```python
from build123d import *

# Parameters (mm, degrees)
SKETCH1_W                       = 9.525
SKETCH1_H                       = 9.525
BOSS_EXTRUDE1_DEPTH             = 9.525
CUT_EXTRUDE2_DEPTH              = 10.525
CUT_EXTRUDE3_DEPTH              = 10.525
F_5_64_0_07813_DIAMETER_HOLE1_D = 1.984502


with BuildPart() as part:
    # Sketch1 → Boss-Extrude1 (new body)
    with BuildSketch(Plane(origin=(0, 0, 0), x_dir=(1, 0, 0), z_dir=(0, 1, 0))):
        with BuildLine():
            Line((-4.138568073, 94.60926025), (4.138568073, 94.60926025))
            ThreePointArc((4.138568073, 94.60926025), (8.245532024, 93.102332324), (10.40323655, 89.29677115))
            Line((10.40323655, 89.29677115), (10.40323655, -5.448440201))
            Line((10.40323655, -5.448440201), (25.4, -29.21573975))
            Line((25.4, -29.21573975), (25.4, -38.74073975))
            Line((25.4, -38.74073975), (28.575, -38.74073975))
            Line((28.575, -38.74073975), (28.575, -83.19073975))
            Line((28.575, -83.19073975), (-28.575, -83.19073975))
            Line((-28.575, -83.19073975), (-28.575, -38.74073975))
            Line((-28.575, -38.74073975), (-25.4, -38.74073975))
            Line((-25.4, -38.74073975), (-25.4, -29.21573975))
            Line((-25.4, -29.21573975), (-10.40323655, -5.448440201))
            Line((-10.40323655, -5.448440201), (-10.40323655, 89.29677115))
            ThreePointArc((-10.40323655, 89.29677115), (-8.245532024, 93.102332324), (-4.138568073, 94.60926025))
        make_face()
        with Locations((0, -65.72823975)):
            Rectangle(SKETCH1_W, SKETCH1_H, mode=Mode.SUBTRACT)
        with Locations((0, 83.49676025)):
            Rectangle(SKETCH1_W, SKETCH1_H, mode=Mode.SUBTRACT)
    extrude(amount=BOSS_EXTRUDE1_DEPTH)

    # Sketch4 → Cut-Extrude2 (cut, through all)
    with BuildSketch(Plane(origin=(0, 9.525, 0), x_dir=(1, 0, 0), z_dir=(0, 1, 0))):
        with BuildLine():
            Line((4.7625, 51.74676025), (4.7625, -14.92823975))
            ThreePointArc((4.7625, -14.92823975), (0, -19.69073975), (-4.7625, -14.92823975))
            Line((-4.7625, -14.92823975), (-4.7625, 51.74676025))
            ThreePointArc((-4.7625, 51.74676025), (0, 56.50926025), (4.7625, 51.74676025))
        make_face()
    extrude(amount=-CUT_EXTRUDE2_DEPTH, mode=Mode.SUBTRACT)

    # Sketch5 → Cut-Extrude3 (cut, through all)
    with BuildSketch(Plane(origin=(0, 9.525, 0), x_dir=(1, 0, 0), z_dir=(0, 1, 0))):
        with BuildLine():
            Line((-22.225, -83.19073975), (22.225, -83.19073975))
            Line((22.225, -83.19073975), (22.225, -81.60323975))
            ThreePointArc((22.225, -81.60323975), (21.760032015, -80.480707734), (20.6375, -80.01573975))
            Line((20.6375, -80.01573975), (-20.6375, -80.01573975))
            ThreePointArc((-20.6375, -80.01573975), (-21.760032015, -80.480707734), (-22.225, -81.60323975))
            Line((-22.225, -81.60323975), (-22.225, -83.19073975))
        make_face()
    extrude(amount=-CUT_EXTRUDE3_DEPTH, mode=Mode.SUBTRACT)

    # 5/64 (0.07813) Diameter Hole1 (through all)
    with Locations(Plane(origin=(0, 9.525, 0), x_dir=(1, 0, 0), z_dir=(0, 1, 0))):
        with Locations((-4.7625, 88.25926025), (4.7625, 88.25926025), (4.7625, 78.73426025), (-4.7625, 78.73426025), (-4.7625, -60.96573975), (4.7625, -60.96573975), (4.7625, -70.49073975), (-4.7625, -70.49073975)):
            Hole(F_5_64_0_07813_DIAMETER_HOLE1_D / 2)


solid = part.part
```
Here's how the part is built. I have some questions about the finished solid (model axes, mm). A direction names the side the tool comes from. Give positions to 0.01 mm unless a question says otherwise; leave off trailing zeros. Order: outer loops, then holes, each group sorted by start corner. A loop starts at its lowest first (then second) coordinate and runs counter-clockwise, first axis right, second up. Notation, with made-up numbers: (79.25, 55.5) -> (121.25, 55.5) arc R13 ccw to (121.25, 66.5) -> close; hole circle Ø2 at (40.25, 12). An arc over 180 degrees is marked (long way). Use CSV: the item, a comma, the result in double quotes. Start each with the question number.
Item 1: Suppose I cut it at B-B (z = -24.5). List the corners of the cut face in (x, y) for me (1 decimal), and give its area (3 significant figures).
Item 2: Thinking about a two-plate mould opening in Z: for faces 4 (the flat face through (-4.762, 5, 66)), 5 (the flat face through (28.575, 5, 61)), 6 (the flat face through (4.762, 5, -19)), 7 (the flat face through (-27, 5, 38.741)), which applies, pulls with the +Z half, pulls with the -Z half, needs draft (parallel to the pull), parting line crosses it, or undercut?
Item 3: If I drill on probe 1 along Z at (x, y) = (-0.5, 3); probe 2 along Z at (x, y) = (1, 6.25); probe 3 along X at (y, z) = (7.5, -17), over which ranges is the centre line in solid material (lowest first)? Write a range as [from, to].
Item 4: Suppose I cut it at A-A (x = 0). List the corners of the cut face in (y, z) for me (3 decimals), and give its area (3 significant figures).
Item 5: Suppose I cut it at D-D (z = 18). List the corners of the cut face in (x, y) for me (3 decimals), and give its area (3 significant figures).
Item 6: I'm going to push flat-ended pins straight in: P1, Ø2, axis at y = 2.5, z = 32, coming from the -X side; P2, Ø1.5, axis at y = 6.5, z = -67, coming from the +X side; P3, Ø1.5, axis at x = -13.5, y = 7, coming from the -Z side. Where does each tip first touch, or does it pass through?
Item 7: On a 3-axis mill with a long thin cutter (end or side, diameter ignored), from which of +Z, -Z, +X, -X, +Y, -Y can I reach the whole of each face in a straight line? I mean faces 1 (the flat face through (10.403, 5, -43)), 2 (the flat face through (0, 5, 60.966)), 3 (the flat face through (-25.4, 5, 34)). Say none if no direction works.
Item 8: Suppose I cut it at C-C (y = 7.5). Give the number of separate pieces and of enclosed holes in the cut face, and give its area (3 significant figures).
Answer block:
1,outline,"(-10.4, 0) -> (-4.8, 0) -> (-4.8, 9.5) -> (-10.4, 9.5) -> close; (4.8, 0) -> (10.4, 0) -> (10.4, 9.5) -> (4.8, 9.5) -> close"
1,area,"107 mm^2"
2,face 4,"undercut"
2,face 5,"needs draft"
2,face 6,"undercut"
2,face 7,"pulls with the -Z half"
3,probe 1,"z = [-94.61, -88.26], [-78.73, -56.48], [19.66, 60.97], [70.49, 80.02]"
3,probe 2,"z = [-94.61, -88.26], [-78.73, -56.4], [19.58, 60.97], [70.49, 80.02]"
3,probe 3,"x = [-10.4, -4.76], [4.76, 10.4]"
4,outline,"(0, -94.609) -> (9.525, -94.609) -> (9.525, -88.259) -> (0, -88.259) -> close; (0, -78.734) -> (9.525, -78.734) -> (9.525, -56.509) -> (0, -56.509) -> close; (0, 19.691) -> (9.525, 19.691) -> (9.525, 60.966) -> (0, 60.966) -> close; (0, 70.491) -> (9.525, 70.491) -> (9.525, 80.016) -> (0, 80.016) -> close"
4,area,"756 mm^2"
5,outline,"(-18.323, 0) -> (-3.639, 0) -> (-3.639, 9.525) -> (-18.323, 9.525) -> close; (3.639, 0) -> (18.323, 0) -> (18.323, 9.525) -> (3.639, 9.525) -> close"
5,area,"280 mm^2"
6,P1,"stops at x = -25.4"
6,P2,"stops at x = 10.4"
6,P3,"stops at z = 9.17"
7,face 1,"-Z, +X, +Y, -Y"
7,face 2,"+Y, -Y"
7,face 3,"-Z, -X, +Y, -Y"
8,separate pieces,"1"
8,enclosed holes,"3"
8,area,"4,890 mm^2"
